The model under review builds one solid part; all positions refer to its coordinate system, in mm. Face numbers are marked on the shaded views. Give positions to 0.01 mm unless a question says otherwise; leave off trailing zeros. Order: outer loops, then holes, each group sorted by start corner. A loop starts at its lowest first (then second) coordinate and runs counter-clockwise, first axis right, second up. Notation, with made-up numbers: (-5, 18.25) - (52, 18.25) arc R28 ccw to (52, 39.25) - close; hole circle Ø7 at (-3.75, -8). An arc over 180 degrees is marked (long way). Put each result on its own line as item: value.
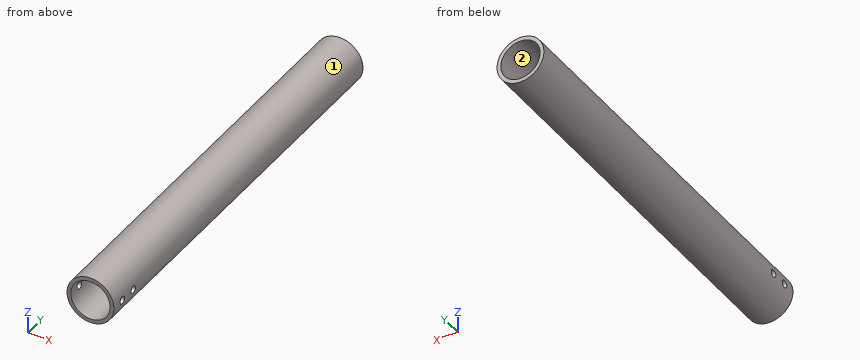
```python
from build123d import *

# Parameters (mm, degrees)
SKETCH_1_R          = 12.5
SKETCH_1_R_2        = 10.5
EXTRUDE_1_DEPTH     = 220
SKETCH_4_R          = 2
CUT_EXTRUDE_1_DEPTH = 100


with BuildPart() as part:
    # Эскиз1 → Вытянуть1 (new body)
    with BuildSketch(Plane(origin=(0, 0, 0), x_dir=(1, 0, 0), z_dir=(0, 1, 0))):
        with Locations(Location((0, 0, 0), (0, 0, 270))):
            Circle(SKETCH_1_R)
        with Locations(Location((0, 0, 0), (0, 0, 270))):
            Circle(SKETCH_1_R_2, mode=Mode.SUBTRACT)
    extrude(amount=EXTRUDE_1_DEPTH)

    # Эскиз4 → Вырез-Вытянуть1 (cut, symmetric)
    with BuildSketch(Plane(origin=(0, 0, 0), x_dir=(0, 0, -1), z_dir=(1, 0, 0))):
        with Locations((0, 17.141022055)):
            Circle(SKETCH_4_R)
        with Locations((0, 7.474896081)):
            Circle(SKETCH_4_R)
    extrude(amount=CUT_EXTRUDE_1_DEPTH, both=True, mode=Mode.SUBTRACT)


solid = part.part
```
(1) Take a section at D-D, the plane y = 75. Write out the cut boundary in (x, z), then the cut area to 3 significant figures.
The answers:
outline: circle Ø25 at (0, 0); hole circle Ø21 at (0, 0)
area: 145 mm^2
(2) Take a section at A-A, the plane x = 0. Write out the cut boundary in (y, z).
The answers:
outline: (0, -12.5) - (220, -12.5) - (220, -10.5) - (0, -10.5) - close; (0, 10.5) - (220, 10.5) - (220, 12.5) - (0, 12.5) - close
(3) Take a section at C-C, the plane z = 8.5. Write out the cut boundary in (x, y).
The answers:
outline: (-9.17, 0) - (-6.16, 0) - (-6.16, 220) - (-9.17, 220) - close; (6.16, 0) - (9.17, 0) - (9.17, 220) - (6.16, 220) - close
(4) Clearance check with flat-ended pins moving along their axes: pin 1 Ø6 at (y, z) = (69, -6.5) entering from +X; pin 2 Ø10 at (x, y) = (10, 165) entering from +Z; pin 3 Ø2 at (y, z) = (84.5, 8) entering from +X; pin 4 Ø12 at (y, z) = (82.5, -5.5) entering from -X. State where each tip first meets the part, or that it passes through.
The answers:
pin 1: x = 12
pin 2: z = 11.46
pin 3: x = 10.36
pin 4: x = -12.5
(5) The part is to be moulded in two halves that separate along X. For the marked faces 1 and 2, say which applies: pulls with the +X half, pulls with the -X half, needs draft (parallel to the pull), parting line crosses it, or undercut.
The answers:
face 1: parting line crosses it
face 2: undercut
(6) Take a section at B-B, the plane z = 0. Write out the cut boundary in (x, y), then the cut area to 3 significant figures.
The answers:
outline: (-12.5, 0) - (-10.5, 0) - (-10.5, 5.47) - (-12.5, 5.47) - close; (-12.5, 9.47) - (-10.5, 9.47) - (-10.5, 15.14) - (-12.5, 15.14) - close; (-12.5, 19.14) - (-10.5, 19.14) - (-10.5, 220) - (-12.5, 220) - close; (10.5, 0) - (12.5, 0) - (12.5, 5.47) - (10.5, 5.47) - close; (10.5, 9.47) - (12.5, 9.47) - (12.5, 15.14) - (10.5, 15.14) - close; (10.5, 19.14) - (12.5, 19.14) - (12.5, 220) - (10.5, 220) - close
area: 848 mm^2
(7) Wall thickness on L1, parallel to Y at x = -11.7, z = 0; L2, parallel to X at y = 168, z = 0; L3, parallel to Z at x = 0.5, y = 120: over which ranges is each line inside the solid? List them lowest first.
The answers:
L1: 0 to 5.47, 9.47 to 15.14, 19.14 to 220
L2: -12.5 to -10.5, 10.5 to 12.5
L3: -12.49 to -10.49, 10.49 to 12.49
